Could you check a few things on this drawing? It's one solid part, dimensions in mm from its lowest x, y, z. A direction names the side the tool comes from. Round coordinates to 2 decimals unless told otherwise and drop trailing zeros. Write each loop counter-clockwise with the first axis right and the second up, starting at its lowest first coordinate (ties: lowest second). Pieces come first, ordered by that corner, then holes. Notation, with made-up numbers: M 21,-3.75 L 37,-3.75 A16 ccw 37,25.25 Z; hole C 31,-38 d3. An arc over 180 degrees is marked long. One line per item, written item: value. Start each with the question number.
(1) I want a section at B-B on y = 140. Please give me the cut outline in (x, z).
(2) Which directions (+Z, -Z, +X, -X, +Y, -Y) give clear straight access to the entire face, cutting with the end or side of a thin tool? Please do the marked faces 4, 5 and 6.
(3) If I drill on L1, parallel to Y at x = 12.5, z = 36.2; L2, parallel to Y at x = 12.5, z = 37.7; L3, parallel to X at y = 140, z = 36.4, over which ranges is the centre line in solid material (lowest first)?
(4) I want a section at C-C on z = 19.5. Please give me the cut outline in (x, y), and give its area (3 significant figures).
(5) Thinking about a two-plate mould opening in Y: for the marked faces 1, 2 and 3, which applies, released by +Y, released by -Y, zero draft, split by the parting line, or undercut?
(6) I'm going to push flat-ended pins straight in: pin 1 Ø2 at (x, z) = (21.5, 12.5) entering from +Y; pin 2 Ø10 at (x, y) = (7, 148.5) entering from -Z; pin 3 Ø3 at (x, y) = (12.5, 15) entering from +Z; pin 4 Ø4 at (x, z) = (6.5, 30.5) entering from +Y. Where does each tip first touch, or does it pass through?
(7) I want a section at D-D on x = 23. Please give me the cut outline in (y, z).
(8) I want a section at A-A on x = 12.5. Please give me the cut outline in (y, z).
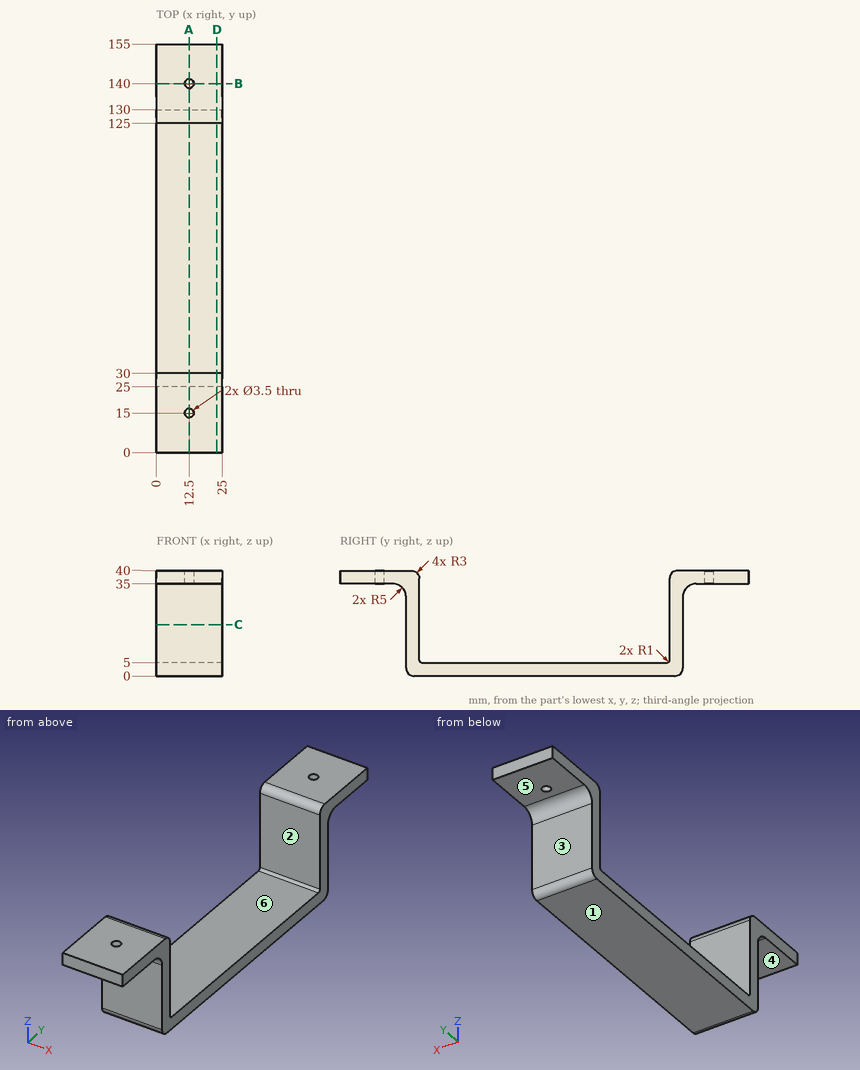
Found:
1. outline: M 0,35 L 10.75,35 L 10.75,40 L 0,40 Z; M 14.25,35 L 25,35 L 25,40 L 14.25,40 Z
2. face 4: -Z, +X, -X, -Y
2. face 5: -Z, +X, -X, +Y
2. face 6: +Z, +X, -X
3. L1: y = 0 to 13.25, 16.75 to 30, 125 to 138.25, 141.75 to 155
3. L2: y = 0 to 13.25, 16.75 to 29.92, 125.08 to 138.25, 141.75 to 155
3. L3: x = 0 to 10.75, 14.25 to 25
4. outline: M 0,25 L 25,25 L 25,30 L 0,30 Z; M 0,125 L 25,125 L 25,130 L 0,130 Z
4. area: 250 mm²
5. face 1: zero draft
5. face 2: undercut
5. face 3: released by +Y
6. pin 1: stops at y = 130
6. pin 2: stops at z = 35
6. pin 3: passes through
6. pin 4: stops at y = 130.67
7. outline: M 0,35 L 20,35 A5 cw 25,30 L 25,3 A3 ccw 28,0 L 127,0 A3 ccw 130,3 L 130,30 A5 cw 135,35 L 155,35 L 155,40 L 128,40 A3 ccw 125,37 L 125,6 A1 cw 124,5 L 31,5 A1 cw 30,6 L 30,37 A3 ccw 27,40 L 0,40 Z
8. outline: M 0,35 L 13.25,35 L 13.25,40 L 0,40 Z; M 16.75,35 L 20,35 A5 cw 25,30 L 25,3 A3 ccw 28,0 L 127,0 A3 ccw 130,3 L 130,30 A5 cw 135,35 L 138.25,35 L 138.25,40 L 128,40 A3 ccw 125,37 L 125,6 A1 cw 124,5 L 31,5 A1 cw 30,6 L 30,37 A3 ccw 27,40 L 16.75,40 Z; M 141.75,35 L 155,35 L 155,40 L 141.75,40 Z
